from build123d import *

# Parameters (mm, degrees)
F0_W     = 15
F0_H     = 10
F1_DEPTH = 2
F2_R     = 2
F3_DEPTH = 2.001
F4_R     = 17.5
F5_DEPTH = 2.001
F6_W     = 15
F6_H     = 10
F7_DEPTH = 8
F8_R     = 2.1
F9_DEPTH = 27.501
F10_R    = 4.99999


# Not quite as in the source:
# - a fillet or chamfer is up to 0.001 mm smaller than in the source, because OpenCascade refuses the exact size


with BuildPart() as f1:
    # F0 (on Top) → F1 (new body)
    with BuildSketch(Plane.XY):
        Polygon((0, 40), (0, 0), (40, 0), (40, 40), (27.5, 40), (12.5, 40), align=None)
        with Locations((20, 45)):
            Rectangle(F0_W, F0_H)
    extrude(amount=F1_DEPTH)

    # F2 (on face) → F3 (cut, through all)
    with BuildSketch(Plane.XY.offset(2)):
        with Locations((4, 36)):
            Circle(F2_R)
        with Locations((36, 36)):
            Circle(F2_R)
        with Locations((4, 4)):
            Circle(F2_R)
        with Locations((36, 4)):
            Circle(F2_R)
    extrude(amount=-F3_DEPTH, mode=Mode.SUBTRACT)

    # F4 (on face) → F5 (cut, through all)
    with BuildSketch(Plane.XY.offset(2)):
        with Locations((20, 20)):
            Circle(F4_R)
    extrude(amount=-F5_DEPTH, mode=Mode.SUBTRACT)

    # F6 (on face) → F7 (join)
    with BuildSketch(Plane(origin=(0, 0, 0), x_dir=(1, 0, 0), z_dir=(0, 0, -1))):
        with Locations((20, -45)):
            Rectangle(F6_W, F6_H)
    extrude(amount=F7_DEPTH)

    # F8 (on face) → F9 (cut, through all)
    with BuildSketch(Plane.YZ.offset(27.5)):
        with Locations((45, -3)):
            Circle(F8_R)
    extrude(amount=-F9_DEPTH, mode=Mode.SUBTRACT)

    # F10 (radius 5 in the source; OpenCascade refuses exactly that, so slightly less here)
    f10_edges = [f1.edges().sort_by_distance(p)[0] for p in [
        (20, 50, -8),
        (20, 40, -8),
    ]]
    fillet(f10_edges, radius=F10_R)


solid = f1.part
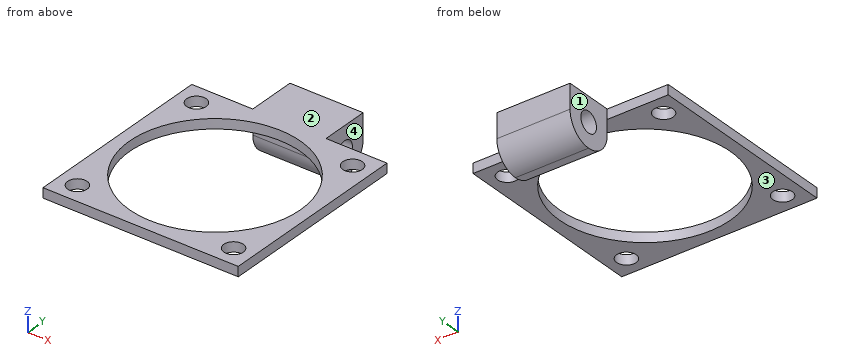
For this review, take the finished solid that the model builds, in its own axes (mm). Face numbers are marked on the shaded views. A direction names the side the tool comes from. Round coordinates to 2 decimals unless told otherwise and drop trailing zeros. Loops run counter-clockwise (first coordinate to the right, second up) from the corner with the lowest first, then second, coordinate; pieces in that order, holes last. Notation, with made-up numbers: (-15.5, 35.25) - (10.5, 35.25) arc R20 cw to (10.5, 53.25) - close; hole circle Ø5 at (68.5, -38.75). An arc over 180 degrees is marked (long way). One line per item, written item: value. Start each with the question number.
Item 1: For L1, parallel to Z at x = 13, y = 45; L2, parallel to Y at x = 20, z = 1.35; L3, parallel to Z at x = 20, y = 38.5, list the stretches that pass through material, from the lowest coordinate up.
Item 2: Take a section at D-D (y = 4). Give the boundary of the cut face in (x, z).
Item 3: Take a section at C-C (z = -1.5). Give the boundary of the cut face in (x, y), plus the area to 3 significant figures.
Item 4: Clearance check with flat-ended pins moving along their axes: pin 1 Ø2 at (x, z) = (8, 0.5) entering from +Y; pin 2 Ø1.5 at (x, z) = (21, -1.5) entering from -Y; pin 3 Ø3 at (x, y) = (12, 40.5) entering from -Z. State where each tip first meets the part, or that it passes through.
Item 5: For the marked faces 1, 2, 3 and 4, list the 3-axis set-ups (+Z, -Z, +X, -X, +Y, -Y) from which the entire face can be reached by the end or side of a thin tool; tool diameter is ignored.
Item 6: Take a section at A-A (y = 20). Give the boundary of the cut face in (x, z).
Item 7: Take a section at B-B (x = 15). State how many separate pieces and enclosed holes the cut face has, plus the area to 3 significant figures.
Answer below:
1. L1: z = -8 to -5.1, -0.9 to 2
1. L2: y = 0 to 2.5, 37.5 to 50
1. L3: z = 0 to 2
2. outline: (0, 0) - (2, 0) - (2, 2) - (0, 2) - close; (6, 0) - (12.91, 0) - (12.91, 2) - (6, 2) - close; (27.09, 0) - (34, 0) - (34, 2) - (27.09, 2) - close; (38, 0) - (40, 0) - (40, 2) - (38, 2) - close
3. outline: (12.5, 40) - (27.5, 40) - (27.5, 43.53) - (12.5, 43.53) - close; (12.5, 46.47) - (27.5, 46.47) - (27.5, 50) - (12.5, 50) - close
3. area: 106 mm2
4. pin 1: stops at y = 40
4. pin 2: stops at y = 40
4. pin 3: stops at z = -6.93
5. face 1: +Z, -Z, -X, +Y
5. face 2: +Z, +X, -X, +Y, -Y
5. face 3: -Z, +X, -X, -Y
5. face 4: +Z, -Z, +X, +Y
6. outline: (0, 0) - (2.5, 0) - (2.5, 2) - (0, 2) - close; (37.5, 0) - (40, 0) - (40, 2) - (37.5, 2) - close
7. separate pieces: 2
7. enclosed holes: 1
7. area: 88.3 mm2
